```python
from build123d import *

# Parameters (mm, degrees)
F0_W      = 90
F0_H      = 10
F1_DEPTH  = 10
F2_T      = -2.5
F3_W      = 7.5
F3_H      = 3
F4_DEPTH  = 2.5
F5_W      = 3
F5_H      = 10
F6_DEPTH  = 7.5
F7_W      = 3
F7_H      = 3
F8_DEPTH  = 3
F9_W      = 3
F9_H      = 2.6932093799
F9_W_2    = 50.1080509275
F10_DEPTH = 2.7
F11_W     = 1.6326196492
F11_H     = 2.7
F12_DEPTH = 2
F13_W     = 2.0434856415
F13_H     = 2.7
F14_DEPTH = 2
F15_W     = 2.5415048003
F15_H     = 10
F16_DEPTH = 1.5


with BuildPart() as f1:
    # F0 (on Top) → F1 (new body)
    with BuildSketch(Plane.XY):
        with Locations((14.7734600306, -2.3407222517)):
            Rectangle(F0_W, F0_H)
    extrude(amount=F1_DEPTH)

    # F2
    f2_openings = [f1.faces().sort_by_distance(p)[0] for p in [
        (59.77346, -2.340722, 5),
        (-30.22654, -2.340722, 5),
    ]]
    offset(amount=F2_T, openings=f2_openings)

    # F3 (on face) → F4 (cut, through all)
    with BuildSketch(Plane.XY.offset(10)):
        with Locations((39.5166127384, -2.3407222517)):
            Rectangle(F3_W, F3_H)
    extrude(amount=-F4_DEPTH, mode=Mode.SUBTRACT)

    # F5 (on face) → F6 (join)
    with BuildSketch(Plane.XY.offset(10)):
        with Locations((25.6160299629, -2.3407222517)):
            Rectangle(F5_W, F5_H)
    extrude(amount=F6_DEPTH)

    # F7 (on face) → F8 (cut)
    with BuildSketch(Plane.XY.offset(17.5)):
        with Locations((25.6160299629, -2.3407222517)):
            Rectangle(F7_W, F7_H)
    extrude(amount=-F8_DEPTH, mode=Mode.SUBTRACT)

    # F9 (on face) → F10 (join)
    with BuildSketch(Plane.XZ.offset(0.8407222517)):
        Polygon((27.1160299629, 14.5), (31.9977998734, 14.5), (39.3753573298, 5.7678297162), (40.6771413982, 6.2636667863), (37.9447564483, 17.1932093799), (27.1160299629, 17.1932093799), align=None)
        with Locations((25.6160299629, 15.84660469)):
            Rectangle(F9_W, F9_H)
        with Locations((-0.9379955009, 15.84660469)):
            Rectangle(F9_W_2, F9_H)
    extrude(amount=F10_DEPTH)

    # F11 (on face) → F12 (join)
    with BuildSketch(Plane(origin=(0, 0, 14.5), x_dir=(1, 0, 0), z_dir=(0, 0, -1))):
        with Locations((23.2997201383, 2.1907222517)):
            Rectangle(F11_W, F11_H)
    extrude(amount=F12_DEPTH)

    # F13 (on face) → F14 (cut)
    with BuildSketch(Plane.XY.offset(17.1932093799)):
        with Locations((34.9011048675, -2.1907222517)):
            Rectangle(F13_W, F13_H)
    extrude(amount=-F14_DEPTH, mode=Mode.SUBTRACT)

    # F15 (on face) → F16 (cut)
    with BuildSketch(Plane(origin=(0, 0, 0), x_dir=(1, 0, 0), z_dir=(0, 0, -1))):
        with Locations((43.5744747519, 2.3407222517)):
            Rectangle(F15_W, F15_H)
    extrude(amount=-F16_DEPTH, mode=Mode.SUBTRACT)


solid = f1.part
```
Design review of the part built by this model. Coordinates are the model's own, in mm. A direction names the side the tool comes from. Give positions to 0.01 mm unless a question says otherwise; leave off trailing zeros. Order: outer loops, then holes, each group sorted by start corner. A loop starts at its lowest first (then second) coordinate and runs counter-clockwise, first axis right, second up. Notation, with made-up numbers: (-8.75, 87.25) -> (-3.75, 87.25) arc R22 ccw to (-3.75, 94.25) -> close; hole circle Ø7 at (-34, 71.25). An arc over 180 degrees is marked (long way). Write item = value, one per line. Start each with the question number.
(1) We need section D-D on y = -2.5. State how many separate pieces and enclosed holes the cut face has, plus the area to 3 significant figures.
(2) For pin 1 (0.6 mm diameter, centred on y = -2.5, z = 16.5, fed in from -X); pin 2 (2 mm diameter, centred on x = 34.5, y = -2.5, fed in from +Z); pin 3 (2.5 mm diameter, centred on x = 0, z = 16, fed in from +Y), all flat-tipped, find the tip position at first contact; note any pin that passes through.
(3) Mouldability with a two-part tool opening along Z and no side actions: class faces 1 (the face through (26, -6, 17.5)), 2 (the face through (14, -4.841, 5)), 3 (the face through (14, 2.659, 5)) as +Z half, -Z half, draft (parallel to the pull), parting line (faces both ways), or undercut.
(4) We need section A-A on x = 13. Write out the cut boundary in (y, z).
(5) To check wall thickness, follow line 1 along Z through (x, y) = (-5, -2.5); line 2 along Y through (x, z) = (35.5, 4.25); line 3 along Z through (x, y) = (54, -3.5). State the ranges of each line that lie inside material, in increasing order.
(6) We need section B-B on z = 3.75. Write out the cut boundary in (x, y).
(7) For faces 4 (the face through (33.879, -2, 16)), 5 (the face through (35.63, -2.17, 10.2)), 6 (the face through (44.845, -2, 1)), list the 3-axis set-ups (+Z, -Z, +X, -X, +Y, -Y) from which the entire face can be reached by the end or side of a thin tool; tool diameter is ignored.
(8) We need section C-C on x = 48.5. Write out the cut boundary in (y, z), plus the area to 3 significant figures.
Numbers:
q1.separate_pieces = 3
q1.enclosed_holes = 0
q1.area = 648 mm^2
q2.pin_1 = -25.99
q2.pin_2 = 17.19
q2.pin_3 = -0.84
q3.face_1 = +Z half
q3.face_2 = undercut
q3.face_3 = draft
q4.outline = (-7.34, 0) -> (2.66, 0) -> (2.66, 10) -> (-7.34, 10) -> close; (-3.54, 14.5) -> (-0.84, 14.5) -> (-0.84, 17.19) -> (-3.54, 17.19) -> close; hole (-4.84, 2.5) -> (0.16, 2.5) -> (0.16, 7.5) -> (-4.84, 7.5) -> close
q5.line_1 = 0 to 2.5, 7.5 to 10, 14.5 to 17.19
q5.line_2 = -7.34 to -4.84, 0.16 to 2.66
q5.line_3 = 0 to 2.5, 7.5 to 10
q6.outline = (-30.23, -7.34) -> (59.77, -7.34) -> (59.77, -4.84) -> (-30.23, -4.84) -> close; (-30.23, 0.16) -> (59.77, 0.16) -> (59.77, 2.66) -> (-30.23, 2.66) -> close
q7.face_4 = +Z, +Y, -Y
q7.face_5 = none
q7.face_6 = -Z, +Y, -Y
q8.outline = (-7.34, 0) -> (2.66, 0) -> (2.66, 10) -> (-7.34, 10) -> close; hole (-4.84, 2.5) -> (0.16, 2.5) -> (0.16, 7.5) -> (-4.84, 7.5) -> close
q8.area = 75.0 mm^2
